Read the model definition and answer for the solid it produces. Units are mm, in the model's axes. Face numbers are marked on the shaded views. Round coordinates to 2 decimals unless told otherwise and drop trailing zeros. Loops run counter-clockwise (first coordinate to the right, second up) from the corner with the lowest first, then second, coordinate; pieces in that order, holes last. Notation, with made-up numbers: M 2.25,6 L 41.25,6 A22 ccw 41.25,29 Z; hole C 9,7.25 d4. An arc over 180 degrees is marked long. Write each question's results on one line, items separated by ' | '.
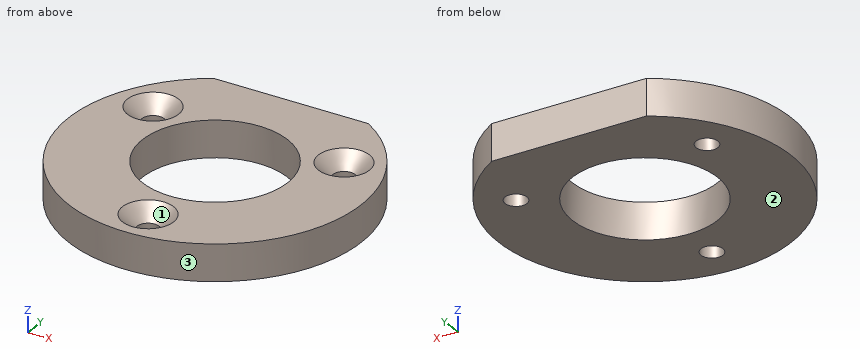
from build123d import *

# Parameters (mm, degrees)
SKETCH1_R           = 9.925
BOSS_EXTRUDE1_DEPTH = 5
SKETCH2_R           = 1.5
CUT_EXTRUDE1_DEPTH  = 29.722813233
CIRPATTERN1_COUNT   = 3
CHAMFER1_SIZE       = 2


with BuildPart() as part:
    # Sketch1 → Boss-Extrude1 (new body)
    with BuildSketch(Plane.XY):
        with BuildLine():
            Line((10.535653753, 17), (-10.535653753, 17))
            ThreePointArc((-10.535653753, 17), (0, -20), (10.535653753, 17))
        make_face()
        Circle(SKETCH1_R, mode=Mode.SUBTRACT)
    extrude(amount=BOSS_EXTRUDE1_DEPTH)

    # Sketch2 → Cut-Extrude1 (cut, through all)
    with BuildSketch(Plane.XY.offset(5)):
        with Locations((0, -15)):
            Circle(SKETCH2_R)
    cut_extrude1 = extrude(amount=-CUT_EXTRUDE1_DEPTH, mode=Mode.SUBTRACT)

    # CirPattern1: Cut-Extrude1 ×3 about axis
    cirpattern1_axis = Axis((0, 0, 0), (0, 0, 1))
    for i in range(1, CIRPATTERN1_COUNT):
        add(cut_extrude1.rotate(cirpattern1_axis, i * 360 / CIRPATTERN1_COUNT), mode=Mode.SUBTRACT)

    # Chamfer1
    chamfer1_edges = [part.edges().sort_by_distance(p)[0] for p in [
        (-1.5, -15, 5),
        (13.740381057, 6.200961894, 5),
        (-12.240381057, 8.799038106, 5),
    ]]
    chamfer(chamfer1_edges, length=CHAMFER1_SIZE)


solid = part.part
Item 1: The part is cut by section D-D (x = 9). Determine the outline of the cut face in (y, z).
Outcome:
outline: M -17.86,0 L -4.18,0 L -4.18,5 L -17.86,5 Z; M 4.18,0 L 17,0 L 17,5 L 4.18,5 Z
Item 2: The part is cut by section A-A (y = 0). Determine the outline of the cut face in (x, z) (3 decimals).
Outcome:
outline: M -20,0 L -9.925,0 L -9.925,5 L -20,5 Z; M 9.925,0 L 20,0 L 20,5 L 9.925,5 Z
Item 3: The part is cut by section B-B (x = 0). Determine the outline of the cut face in (y, z) (3 decimals).
Outcome:
outline: M -20,0 L -16.5,0 L -16.5,3 L -18.5,5 L -20,5 Z; M -13.5,0 L -9.925,0 L -9.925,5 L -11.5,5 L -13.5,3 Z; M 9.925,0 L 17,0 L 17,5 L 9.925,5 Z
Item 4: Straight lines are drawn through the part: line 1 (Y direction, x = 0, z = 2.25) (3 decimals); line 2 (X direction, y = 5.5, z = 3.75); line 3 (Y direction, x = 0.5, z = 1.8). For each, find the intervals that lie inside material, in ascending order.
Outcome:
line 1: y = -20 to -16.5, -13.5 to -9.925, 9.925 to 17 | line 2: x = -19.23 to -14.02, -11.96 to -8.26, 8.26 to 11.96, 14.02 to 19.23 | line 3: y = -19.99 to -16.41, -13.59 to -9.91, 9.91 to 17
Item 5: The mould has two halves that part along X. Classify the marked faces 1, 2 and 3: pulls with the +X half, pulls with the -X half, needs draft (parallel to the pull), parting line crosses it, or undercut.
Outcome:
face 1: undercut | face 2: needs draft | face 3: parting line crosses it
Item 6: Flat-ended cylindrical pins translate along their axes: pin 1 (2 mm diameter, centred on x = -12.5, y = 7, fed in from +Z); pin 2 (3 mm diameter, centred on y = 10, z = 1, fed in from +X); pin 3 (1.5 mm diameter, centred on y = -11.5, z = 2, fed in from +X). Find the tip coordinate at first contact, or state that the pin passes through.
Outcome:
pin 1: stops at z = 3.2 | pin 2: stops at x = 18.1 | pin 3: stops at x = 16.87
Item 7: The part is cut by section C-C (y = 7.5). Determine the outline of the cut face in (x, z), plus the area to 3 significant figures.
Outcome:
outline: M -18.54,0 L -14.49,0 L -14.49,3 L -16.49,5 L -18.54,5 Z; M -11.49,0 L -6.5,0 L -6.5,5 L -9.49,5 L -11.49,3 Z; M 6.5,0 L 11.49,0 L 11.49,3 L 9.49,5 L 6.5,5 Z; M 14.49,0 L 18.54,0 L 18.54,5 L 16.49,5 L 14.49,3 Z | area: 82.4 mm2
